from build123d import *

# Parameters (mm, degrees)
CROQUIS1_W              = 32.5
CROQUIS1_H              = 20.5
SALIENTE_EXTRUIR1_DEPTH = 1
CROQUIS2_R              = 8.4
SALIENTE_EXTRUIR2_DEPTH = 9.5
CROQUIS3_W              = 2.5
CROQUIS3_H              = 10.77685143
SALIENTE_EXTRUIR3_DEPTH = 5.5
CROQUIS4_W              = 10.77685143
CROQUIS4_H              = 1
SALIENTE_EXTRUIR4_DEPTH = 6
CROQUIS5_W              = 3.536132023
CROQUIS5_H              = 3.536132023
SALIENTE_EXTRUIR5_DEPTH = 5
CROQUIS7_R              = 5.1
CORTAR_EXTRUIR1_DEPTH   = 1
REDONDEO1_R             = 1
CROQUIS8_W              = 2.533189813
CROQUIS8_H              = 1
CROQUIS8_W_2            = 2.4671066
CROQUIS8_W_3            = 1.475858413
CORTAR_EXTRUIR2_DEPTH   = 12
REDONDEO2_R             = 0.5


with BuildPart() as part:
    # Croquis1 → Saliente-Extruir1 (new body)
    with BuildSketch(Plane(origin=(0, 0, 0), x_dir=(1, 0, 0), z_dir=(0, 1, 0))):
        with Locations((16.25, 10.25)):
            Rectangle(CROQUIS1_W, CROQUIS1_H)
    extrude(amount=SALIENTE_EXTRUIR1_DEPTH)

    # Croquis2 → Saliente-Extruir2 (add)
    with BuildSketch(Plane(origin=(0, 1, 0), x_dir=(1, 0, 0), z_dir=(0, 1, 0))):
        with Locations(Location((14, 10.3, 0), (0, 0, 270))):
            Circle(CROQUIS2_R)
    extrude(amount=SALIENTE_EXTRUIR2_DEPTH)

    # Croquis3 → Saliente-Extruir3 (add)
    with BuildSketch(Plane.XZ):
        with Locations((31.25, -10.213198871)):
            Rectangle(CROQUIS3_W, CROQUIS3_H)
    extrude(amount=SALIENTE_EXTRUIR3_DEPTH)

    # Croquis4 → Saliente-Extruir4 (add)
    with BuildSketch(Plane(origin=(32.5, 0, 0), x_dir=(0, 0, -1), z_dir=(1, 0, 0))):
        with Locations((10.213198871, -5)):
            Rectangle(CROQUIS4_W, CROQUIS4_H)
    extrude(amount=SALIENTE_EXTRUIR4_DEPTH)

    # Croquis5 → Saliente-Extruir5 (add)
    with BuildSketch(Plane.XZ):
        with Locations((25.43823104, -2.55154591)):
            Rectangle(CROQUIS5_W, CROQUIS5_H)
    extrude(amount=SALIENTE_EXTRUIR5_DEPTH)

    # Croquis7 → Cortar-Extruir1 (cut)
    with BuildSketch(Plane(origin=(0, 10.5, 0), x_dir=(1, 0, 0), z_dir=(0, 1, 0))):
        with Locations(Location((14, 10.3, 0), (0, 0, 270))):
            Circle(CROQUIS7_R)
    extrude(amount=-CORTAR_EXTRUIR1_DEPTH, mode=Mode.SUBTRACT)

    # Redondeo1
    redondeo1_edges = [part.edges().sort_by_distance(p)[0] for p in [
        (14, 10.5, -18.7),
    ]]
    fillet(redondeo1_edges, radius=REDONDEO1_R)

    # Croquis8 → Cortar-Extruir2 (cut)
    with BuildSketch(Plane(origin=(38.5, 0, 0), x_dir=(0, 0, -1), z_dir=(1, 0, 0))):
        with Locations((7.06995271, -5)):
            Rectangle(CROQUIS8_W, CROQUIS8_H)
        with Locations((10.759598741, -5)):
            Rectangle(CROQUIS8_W_2, CROQUIS8_H)
        with Locations((13.810440385, -5)):
            Rectangle(CROQUIS8_W_3, CROQUIS8_H)
    extrude(amount=-CORTAR_EXTRUIR2_DEPTH, mode=Mode.SUBTRACT)

    # Redondeo2
    redondeo2_edges = [part.edges().sort_by_distance(p)[0] for p in [
        (30, -5.5, -5.31406548),
        (30, -5.5, -8.931296528),
        (30, -5.5, -12.53283161),
        (30, -5.5, -15.074997088),
    ]]
    fillet(redondeo2_edges, radius=REDONDEO2_R)


solid = part.part
Check sheet for the modelled part. Datum: model origin and axes. Units: mm. A direction names the side the tool comes from. Round coordinates to 2 decimals unless told otherwise and drop trailing zeros. Write each loop counter-clockwise with the first axis right and the second up, starting at its lowest first coordinate (ties: lowest second). Pieces come first, ordered by that corner, then holes. Notation, with made-up numbers: (-0.5, -9.75) -> (56.5, -9.75) arc R22 cw to (56.5, 22.25) -> close; hole circle Ø8 at (-19, 8.25). An arc over 180 degrees is marked (long way). Answer as CSV lines item,"result". Start each with the question number.
1) Section check A-A on y = -3. Enter the section's corners in (x, z).
2) Section check B-B on z = -10.3. Enter the section's corners in (x, y), and give its area (3 significant figures).
3) Tool access check on faces 1 (the flat face through (32, -3, -15.602)), 2 (the flat face through (32, -3, -4.825)), 3 (the flat face through (35.5, -4.5, -12.5)). Record the directions out of +Z, -Z, +X, -X, +Y, -Y that give a thin tool (end or side, any length) a straight path to the whole face; none if there is none.
4) Release check for a two-part mould opening along Z. For faces 4 (the flat face through (38.5, -5, -9)), 5 (the flat face through (34, -5, -11.993)), 6 (the flat face through (31, -4.5, -7)), 7 (the flat face through (25, -2, -4.32)) record: pulls with the +Z half, pulls with the -Z half, needs draft (parallel to the pull), parting line crosses it, or undercut.
5) Section check D-D on y = 3.75. Enter the section's corners in (x, z), and give its area (3 significant figures).
6) Go/stop test with flat-tipped pins: P1, Ø1.5, axis at y = -3, z = -9.5, coming from the -X side; P2, Ø4, axis at y = -2.5, z = -2.5, coming from the +X side; P3, Ø8, axis at x = 21.5, y = 7, coming from the +Z side. Record where each tip stops, or that it passes through.
7) Material ranges on line 1 (Y direction, x = 15, z = -10.75); line 2 (Y direction, x = 23.5, z = -15.25); line 3 (X direction, y = 9.85, z = -10.3), recorded low to high. Write a range as from..to.
8) Section check C-C on x = 14. Enter the section's corners in (y, z).
Found:
1,outline,"(23.67, -4.32) -> (27.21, -4.32) -> (27.21, -0.78) -> (23.67, -0.78) -> close; (30, -15.6) -> (32.5, -15.6) -> (32.5, -4.82) -> (30, -4.82) -> close"
2,outline,"(0, 0) -> (30, 0) -> (30, -4.5) -> (32.5, -4.5) -> (32.5, 1) -> (22.4, 1) -> (22.4, 9.5) arc R1 ccw to (21.4, 10.5) -> (19.1, 10.5) -> (19.1, 9.5) -> (8.9, 9.5) -> (8.9, 10.5) -> (6.6, 10.5) arc R1 ccw to (5.6, 9.5) -> (5.6, 1) -> (0, 1) -> close"
2,area,"193 mm^2"
3,face 1,"-Z, +X, -X, -Y"
3,face 2,"+Z, +X, -X, -Y"
3,face 3,"+Z, -Z, +X, +Y"
4,face 4,"needs draft"
4,face 5,"undercut"
4,face 6,"undercut"
4,face 7,"pulls with the -Z half"
5,outline,"circle Ø16.8 at (14, -10.3)"
5,area,"222 mm^2"
6,P1,"stops at x = 30"
6,P2,"stops at x = 27.21"
6,P3,"stops at z = -2.66"
7,line 1,"y = 0..9.5"
7,line 2,"y = 0..1"
7,line 3,"x = 5.66..8.9, 19.1..22.34"
8,outline,"(0, -20.5) -> (1, -20.5) -> (1, -18.7) -> (9.5, -18.7) arc R1 ccw to (10.5, -17.7) -> (10.5, -15.4) -> (9.5, -15.4) -> (9.5, -5.2) -> (10.5, -5.2) -> (10.5, -2.9) arc R1 ccw to (9.5, -1.9) -> (1, -1.9) -> (1, 0) -> (0, 0) -> close"
